from build123d import *

# Parameters (mm, degrees)
SKETCH1_W               = 46
SKETCH1_H               = 24.5
BODY_DEPTH              = 31
SKETCH3_W               = 42
SKETCH3_H               = 20.5
SERVO_HOLE_DEPTH        = 29
SKETCH6_R               = 4
BOSS_EXTRUDE3_DEPTH     = 8
BOSS_EXTRUDE4_DEPTH     = 31
CUT_EXTRUDE3_DEPTH      = 2
CUT_EXTRUDE3_DEPTH_BACK = 29
CUT_EXTRUDE4_DEPTH      = 3
CUT_EXTRUDE5_DEPTH      = 93.790422458
CUT_EXTRUDE5_DEPTH_BACK = 93.790422458
SKETCH11_R              = 1.5
SKETCH12_R              = 4.5
CUT_EXTRUDE6_DEPTH      = 6
SKETCH13_R              = 5
CUT_EXTRUDE7_DEPTH      = 2


with BuildPart() as part:
    # Sketch1 → Body (new body)
    with BuildSketch(Plane(origin=(0, 0, 0), x_dir=(1, 0, 0), z_dir=(0, 1, 0))):
        Rectangle(SKETCH1_W, SKETCH1_H)
    extrude(amount=BODY_DEPTH)

    # Sketch3 → Servo Hole (cut)
    with BuildSketch(Plane(origin=(0, 0, 0), x_dir=(1, 0, 0), z_dir=(0, 1, 0))):
        Rectangle(SKETCH3_W, SKETCH3_H)
    extrude(amount=SERVO_HOLE_DEPTH, mode=Mode.SUBTRACT)

    # Sketch6 → Boss-Extrude3 (add)
    with BuildSketch(Plane(origin=(0, 31, 0), x_dir=(1, 0, 0), z_dir=(0, 1, 0))):
        with Locations(Location((10.5, 0, 0), (0, 0, 90))):
            Circle(SKETCH6_R)
    extrude(amount=BOSS_EXTRUDE3_DEPTH)

    # Sketch8 → Boss-Extrude4 (add)
    with BuildSketch(Plane.XZ):
        Polygon((-23, 12.25), (-24.5, 13.75), (-24.5, 63.75), (-30.5, 63.75), (-30.5, 11.264718626), (-23, 3.764718626), align=None)
        Polygon((24.5, 63.75), (24.5, 13.75), (23, 12.25), (23, 3.764718626), (30.5, 11.264718626), (30.5, 63.75), align=None)
    extrude(amount=-BOSS_EXTRUDE4_DEPTH)

    # Sketch5 → Cut-Extrude3 (cut, two sides: drawn at the far end of the back side and taken through both)
    with BuildSketch(Plane.ZY.offset(-23).offset(-CUT_EXTRUDE3_DEPTH_BACK)):
        Polygon((-6, 27), (6, 27), (6, 22), (4.25, 22), (4.25, 2), (-4.25, 2), (-4.25, 22), (-6, 22), align=None)
    extrude(amount=CUT_EXTRUDE3_DEPTH + CUT_EXTRUDE3_DEPTH_BACK, mode=Mode.SUBTRACT)

    # Sketch10 → Cut-Extrude4 (cut)
    with BuildSketch(Plane(origin=(-24.5, 0, 0), x_dir=(0, 0, -1), z_dir=(1, 0, 0))):
        with BuildLine():
            Line((-32.75, 12.5), (-49.75, 9))
            ThreePointArc((-49.75, 9), (-56.25, 15.5), (-49.75, 22))
            Line((-49.75, 22), (-32.75, 18.5))
            ThreePointArc((-32.75, 18.5), (-29.75, 15.5), (-32.75, 12.5))
        make_face()
    extrude(amount=-CUT_EXTRUDE4_DEPTH, mode=Mode.SUBTRACT)

    # Sketch11 → Cut-Extrude5 (cut, two sides: drawn at the far end of the back side and taken through both)
    with BuildSketch(Plane(origin=(-24.5, 0, 0), x_dir=(0, 0, -1), z_dir=(1, 0, 0)).offset(-CUT_EXTRUDE5_DEPTH_BACK)):
        with Locations((-49.75, 15.5)):
            Circle(SKETCH11_R)
    extrude(amount=CUT_EXTRUDE5_DEPTH + CUT_EXTRUDE5_DEPTH_BACK, mode=Mode.SUBTRACT)

    # Sketch12 → Cut-Extrude6 (cut)
    with BuildSketch(Plane(origin=(30.5, 0, 0), x_dir=(0, 0, -1), z_dir=(1, 0, 0))):
        with Locations((-49.75, 15.5)):
            Circle(SKETCH12_R)
    extrude(amount=-CUT_EXTRUDE6_DEPTH, mode=Mode.SUBTRACT)

    # Sketch13 → Cut-Extrude7 (cut)
    with BuildSketch(Plane.ZY.offset(30.5)):
        with Locations((49.75, 15.5)):
            Circle(SKETCH13_R)
    extrude(amount=-CUT_EXTRUDE7_DEPTH, mode=Mode.SUBTRACT)


solid = part.part
Model file for the job. Use its own axes, mm. A direction names the side the tool comes from. Coordinates: 2 decimals unless noted, no trailing zeros. Order: outer loops, then holes, each group sorted by start corner. A loop starts at its lowest first (then second) coordinate and runs counter-clockwise, first axis right, second up. Notation, with made-up numbers: M 67.5,88.5 L 96.5,88.5 A20 ccw 96.5,95.5 Z; hole C 37.5,56 d1. An arc over 180 degrees is marked long. Return JSON: item names as keys, results as strings.
1. Tool access for faces 1 (the face through (22, 12, -4.25)), 2 (the face through (-25.98, 15.36, 56.25)), 3 (the face through (21, 14, 5)), 4 (the face through (-29.51, 12.46, 45.78)): list every direction of +Z, -Z, +X, -X, +Y, -Y with a clear straight run to the whole face (end or side of a thin tool).
Ans:
{"face 1": "+X", "face 2": "none", "face 3": "-Y", "face 4": "-X"}
2. Flat gauge pins, fed straight in: pin 1 (6 mm diameter, centred on y = 14, z = -4.5, fed in from -X); pin 2 (1.5 mm diameter, centred on y = 24.5, z = 8.5, fed in from +X); pin 3 (15.5 mm diameter, centred on x = -6, y = 18.5, fed in from +Z); pin 4 (8 mm diameter, centred on y = 15.5, z = 51.5, fed in from -X). Where does each tip first touch, or does it go through?
Ans:
{"pin 1": "x = -23", "pin 2": "x = 28.49", "pin 3": "z = 12.25", "pin 4": "x = -30.5"}
3. Saw through at B-B (x = 10.5). Give the cut face in (y, z), and give its area (3 significant figures).
Ans:
{"outline": "M 0,-12.25 L 31,-12.25 L 31,-4 L 39,-4 L 39,4 L 31,4 L 31,12.25 L 0,12.25 L 0,10.25 L 29,10.25 L 29,-10.25 L 0,-10.25 Z", "area": "229 mm^2"}
4. Saw through at A-A (z = 0). Give the cut face in (x, y).
Ans:
{"outline": "M -23,0 L -21,0 L -21,29 L 21,29 L 21,27 L 23,27 L 23,31 L 14.5,31 L 14.5,39 L 6.5,39 L 6.5,31 L -23,31 Z; M 21,0 L 23,0 L 23,2 L 21,2 Z"}
5. Saw through at C-C (y = 7.5). Give the cut face in (x, z).
Ans:
{"outline": "M -30.5,11.26 L -23,3.76 L -23,-12.25 L 23,-12.25 L 23,-4.25 L 21,-4.25 L 21,-10.25 L -21,-10.25 L -21,10.25 L 21,10.25 L 21,4.25 L 23.49,4.25 L 30.5,11.26 L 30.5,63.75 L 24.5,63.75 L 24.5,13.75 L 23,12.25 L -23,12.25 L -24.5,13.75 L -24.5,63.75 L -30.5,63.75 Z"}
6. Saw through at D-D (x = -26). Give the cut face in (y, z), and give its area (3 significant figures).
Ans:
{"outline": "M 0,6.76 L 31,6.76 L 31,63.75 L 0,63.75 Z; hole M 9,49.75 L 12.5,32.75 A3 ccw 18.5,32.75 L 22,49.75 A6.5 ccw Z", "area": "1,520 mm^2"}
7. Drill centre lines: probe 1 along Z at (x, y) = (18, 3.5); probe 2 along X at (y, z) = (5, 41); probe 3 along X at (y, z) = (18, 33). Where is each one in solid material? Low to high.
Ans:
{"probe 1": "-12.25 to -10.25, 10.25 to 12.25", "probe 2": "-30.5 to -24.5, 24.5 to 30.5", "probe 3": "-30.5 to -27.5, 24.5 to 30.5"}
8. Pull direction Z, two halves, no side cores. Call faces 5 (the face through (0, 31, 9)), 6 (the face through (-25.979, 10.774, 41.131)), 7 (the face through (0, 15, -12.25)): +Z half, -Z half, draft (parallel to the pull), parting line (faces both ways), or undercut.
Ans:
{"face 5": "draft", "face 6": "undercut", "face 7": "-Z half"}
